Input: part model. Units: mm. Frame: model coordinates. A direction names the side the tool comes from. Give positions to 0.01 mm unless a question says otherwise; leave off trailing zeros. Loops run counter-clockwise (first coordinate to the right, second up) from the corner with the lowest first, then second, coordinate; pieces in that order, holes last. Notation, with made-up numbers: M 86.5,28.5 L 142.5,28.5 A8 cw 142.5,32.5 Z; hole C 80.5,3 d10. An arc over 180 degrees is marked long. Use CSV: the item, a comma, the result in double quotes. Start each with the question number.
from build123d import *

# Parameters (mm, degrees)
EXTRUDE_1_DEPTH     = 75
FILLET_1_R          = 1
FILLET_2_R          = 1
SKETCH_2_R          = 1.6
SKETCH_2_R_2        = 1.617183579
CUT_EXTRUDE_1_DEPTH = 14


with BuildPart() as part:
    # 草图1 → 凸台-拉伸1 (new body)
    with BuildSketch(Plane.XY):
        Polygon((0, 0), (9, 0), (9, -4), (7.2, -5.529317293), (9, -7.647909697), (0, -7.647909697), (1.8, -5.529317293), (0, -4), align=None)
    extrude(amount=EXTRUDE_1_DEPTH)

    # 圆角1
    fillet_1_edges = [part.edges().sort_by_distance(p)[0] for p in [
        (0, 0, 37.5),
        (9, 0, 37.5),
    ]]
    fillet(fillet_1_edges, radius=FILLET_1_R)

    # 圆角2
    fillet_2_edges = [part.edges().sort_by_distance(p)[0] for p in [
        (9, -4, 37.5),
        (0, -4, 37.5),
    ]]
    fillet(fillet_2_edges, radius=FILLET_2_R)

    # 草图2 → 切除-拉伸1 (cut)
    with BuildSketch(Plane.XZ.offset(7.647909697)):
        with Locations(Location((4.5, 68, 0), (0, 0, 270))):
            Circle(SKETCH_2_R)
        with Locations(Location((4.5, 48, 0), (0, 0, 270))):
            Circle(SKETCH_2_R)
        with Locations(Location((4.5, 28, 0), (0, 0, 270))):
            Circle(SKETCH_2_R)
        with Locations(Location((4.5, 8, 0), (0, 0, 270))):
            Circle(SKETCH_2_R_2)
    extrude(amount=-CUT_EXTRUDE_1_DEPTH, mode=Mode.SUBTRACT)


solid = part.part
Item 1: Section B-B (z = 28). Output: boundary loops of the cut face in (x, y), then the cut area to 3 significant figures.
Item 2: Section C-C (y = -7). Output: boundary loops of the cut face in (x, z).
Item 3: Mould query, pull axis X, two halves, no side actions, for faces 1 (the flat face through (4, 0, 37)), 2 (the cylindrical face through (4.981, -3.877, 66.474)), 3 (the cylindrical face through (4.981, -3.877, 46.474)), 4 (the flat face through (0, -2, 37)). Classes: +X half, -X half, draft (parallel to the pull), parting line (faces both ways), or undercut.
Item 4: Material intervals for line 1 (Z direction, x = 5.25, y = -6); line 2 (Z direction, x = 5.75, y = -1.5); line 3 (X direction, y = -2.5, z = 68), sorted ascending.
Item 5: Section D-D (z = 8). Output: boundary loops of the cut face in (x, y).
Item 6: Set-up query: faces 5 (the flat face through (5, -7.648, 37)), 6 (the flat face through (7.93, -4.91, 36.98)), 7 (the flat face through (1.086, -4.923, 36.975)). Return all of +Z, -Z, +X, -X, +Y, -Y with unobstructed straight access to the full face (end or side cutting, diameter ignored); none if empty.
Item 7: Section A-A (x = 4.5). Output: boundary loops of the cut face in (y, z), then the cut area to 3 significant figures.
Recorded:
1,outline,"M 0,-7.65 L 2.9,-7.65 L 2.9,0 L 1,0 A1 ccw 0,-1 L 0,-3.54 A1 ccw 0.35,-4.3 L 1.8,-5.53 Z; M 6.1,-7.65 L 9,-7.65 L 7.2,-5.53 L 8.65,-4.3 A1 ccw 9,-3.54 L 9,-1 A1 ccw 8,0 L 6.1,0 Z"
1,area,"37.3 mm²"
2,outline,"M 0.55,0 L 8.45,0 L 8.45,75 L 0.55,75 Z; hole C 4.5,8 d3.23; hole C 4.5,28 d3.2; hole C 4.5,48 d3.2; hole C 4.5,68 d3.2"
3,face 1,"draft"
3,face 2,"undercut"
3,face 3,"undercut"
3,face 4,"-X half"
4,line 1,"0 to 6.57, 9.43 to 26.59, 29.41 to 46.59, 49.41 to 66.59, 69.41 to 75"
4,line 2,"0 to 6.97, 9.03 to 27, 29 to 47, 49 to 67, 69 to 75"
4,line 3,"0 to 2.9, 6.1 to 9"
5,outline,"M 0,-7.65 L 2.88,-7.65 L 2.88,0 L 1,0 A1 ccw 0,-1 L 0,-3.54 A1 ccw 0.35,-4.3 L 1.8,-5.53 Z; M 6.12,-7.65 L 9,-7.65 L 7.2,-5.53 L 8.65,-4.3 A1 ccw 9,-3.54 L 9,-1 A1 ccw 8,0 L 6.12,0 Z"
6,face 5,"+Z, -Z, +X, -X, -Y"
6,face 6,"+Z, -Z, +X"
6,face 7,"+Z, -Z, -X"
7,outline,"M -7.65,0 L 0,0 L 0,6.38 L -7.65,6.38 Z; M -7.65,9.62 L 0,9.62 L 0,26.4 L -7.65,26.4 Z; M -7.65,29.6 L 0,29.6 L 0,46.4 L -7.65,46.4 Z; M -7.65,49.6 L 0,49.6 L 0,66.4 L -7.65,66.4 Z; M -7.65,69.6 L 0,69.6 L 0,75 L -7.65,75 Z"
7,area,"475 mm²"
